```python
from build123d import *

# Parameters (mm, degrees)
F0_W     = 60
F0_H     = 60
F0_R     = 11.05
F1_DEPTH = 4
F2_D     = 3.2
F3_D     = 6
F4_SIZE  = 1


with BuildPart() as f1:
    # F0 (on Top) → F1 (new body)
    with BuildSketch(Plane.XY):
        Rectangle(F0_W, F0_H)
        Circle(F0_R, mode=Mode.SUBTRACT)
    extrude(amount=F1_DEPTH)

    # F2 (through all)
    with Locations(Plane(origin=(0, 0, 0), x_dir=(1, 0, 0), z_dir=(0, 0, -1))):
        with Locations((15.5, 15.5), (15.5, -15.5), (-15.5, -15.5), (-15.5, 15.5)):
            Hole(F2_D / 2)

    # F3 (through all)
    with Locations(Plane(origin=(0, 0, 0), x_dir=(1, 0, 0), z_dir=(0, 0, -1))):
        with Locations((-25, -25), (25, -25), (25, 25), (-25, 25)):
            Hole(F3_D / 2)

    # F4
    f4_edges = [f1.edges().sort_by_distance(p)[0] for p in [
        (-11.05, 0, 4),
        (0, -30, 4),
        (-30, 0, 4),
        (0, 30, 4),
        (30, 0, 4),
    ]]
    chamfer(f4_edges, length=F4_SIZE)


solid = f1.part
```
Model file for the job. Use its own axes, mm. Round coordinates to 2 decimals unless told otherwise and drop trailing zeros. Write each loop counter-clockwise with the first axis right and the second up, starting at its lowest first coordinate (ties: lowest second). Pieces come first, ordered by that corner, then holes. Notation, with made-up numbers: M 63.5,-30 L 97.5,-30 A26 ccw 97.5,4 Z; hole C 1,81 d3. An arc over 180 degrees is marked long. Put each result on its own line as item: value.
Item 1: Probe L1, parallel to X at y = 15.5, z = 2.1; L2, parallel to X at y = 25, z = 0.9. List the from-to ranges inside material, lowest first. Write a range as from..to.
Responses:
L1: -30..-17.1, -13.9..13.9, 17.1..30
L2: -30..-28, -22..22, 28..30
Item 2: Cut at C-C (z = 1.6). State how many separate pieces and enclosed holes the cut face has, and give its area (3 significant figures).
Responses:
separate pieces: 1
enclosed holes: 9
area: 3,070 mm²
Item 3: Flat gauge pins, fed straight in: P1, Ø4, axis at x = 15.5, y = -15.5, coming from the -Z side; P2, Ø5.5, axis at x = 25, y = -25, coming from the -Z side. Where does each tip first touch, or does it go through?
Responses:
P1: z = 0
P2: through
Item 4: Cut at A-A (x = 15.5). List the corners of the cut face in (y, z), and give its area (3 significant figures).
Responses:
outline: M -30,0 L -17.1,0 L -17.1,4 L -29,4 L -30,3 Z; M -13.9,0 L 13.9,0 L 13.9,4 L -13.9,4 Z; M 17.1,0 L 30,0 L 30,3 L 29,4 L 17.1,4 Z
area: 213 mm²
Item 5: Mould opens along X. For faces 1 (the flat face through (-30, 0, 1)), 2 (the cylindrical face through (-22, 25, 2)), 3 (the flat face through (0, 14, 0)) say: +X half, -X half, draft (parallel to the pull), parting line (faces both ways), or undercut.
Responses:
face 1: -X half
face 2: undercut
face 3: draft
